from build123d import *

# Parameters (mm, degrees)
SKETCH1_R           = 42.672
SKETCH1_R_2         = 38.862
BOSS_EXTRUDE1_DEPTH = 29.21
SKETCH2_R           = 42.672
SKETCH2_R_2         = 14.478
BOSS_EXTRUDE2_DEPTH = 7.62
SKETCH3_R           = 2.159
CUT_EXTRUDE1_DEPTH  = 43.672
CIRPATTERN1_COUNT   = 4


with BuildPart() as part:
    # Sketch1 → Boss-Extrude1 (new body)
    with BuildSketch(Plane(origin=(0, 0, 0), x_dir=(1, 0, 0), z_dir=(0, 1, 0))):
        Circle(SKETCH1_R)
        Circle(SKETCH1_R_2, mode=Mode.SUBTRACT)
    extrude(amount=BOSS_EXTRUDE1_DEPTH)

    # Sketch2 → Boss-Extrude2 (add)
    with BuildSketch(Plane(origin=(0, 29.21, 0), x_dir=(1, 0, 0), z_dir=(0, 1, 0))):
        Circle(SKETCH2_R)
        Circle(SKETCH2_R_2, mode=Mode.SUBTRACT)
    extrude(amount=BOSS_EXTRUDE2_DEPTH)

    # Sketch3 → Cut-Extrude1 (cut, symmetric)
    with BuildSketch(Plane.XY):
        with Locations((0, 3.937)):
            Circle(SKETCH3_R)
    cut_extrude1 = extrude(amount=CUT_EXTRUDE1_DEPTH, both=True, mode=Mode.SUBTRACT)

    # CirPattern1: Cut-Extrude1 ×4 about axis
    cirpattern1_axis = Axis((0, 29.21, 0), (0, -1, 0))
    for i in range(1, CIRPATTERN1_COUNT):
        add(cut_extrude1.rotate(cirpattern1_axis, i * 360 / CIRPATTERN1_COUNT), mode=Mode.SUBTRACT)


solid = part.part
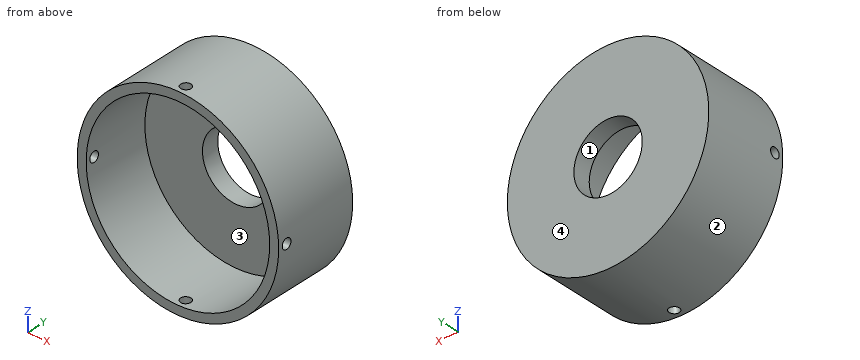
Model file for the job. Use its own axes, mm. Face numbers are marked on the shaded views. Give positions to 0.01 mm unless a question says otherwise; leave off trailing zeros. Loops run counter-clockwise (first coordinate to the right, second up) from the corner with the lowest first, then second, coordinate; pieces in that order, holes last.
1) Saw through at C-C (z = 12). Write the cut outline in (x, y), plus the area to 3 significant figures.
2) Wall check: line 1 (Y direction, x = 0, z = -39.75); line 2 (Z direction, x = 0, y = 34.5); line 3 (Z direction, x = 0, y = 22). Give the ranges that are in metal, low to high.
3) Saw through at A-A (z = 0). Write the cut outline in (x, y).
4) Flat gauge pins, fed straight in: pin 1 Ø5.5 at (x, y) = (0, 3.937) entering from -Z; pin 2 Ø10 at (x, y) = (-22, 8) entering from +Z; pin 3 Ø6 at (x, z) = (-32, -10.5) entering from -Y; pin 4 Ø8 at (x, y) = (28.5, 11) entering from +Z. Where does each tip first touch, or does it go through?
5) Pull direction X, two halves, no side cores. Call the marked faces 1, 2, 3 and 4: +X half, -X half, draft (parallel to the pull), parting line (faces both ways), or undercut.
6) Saw through at B-B (x = 0). Write the cut outline in (y, z), plus the area to 3 significant figures.
7) Saw through at D-D (y = 27.5). Write the cut outline in (x, z), plus the area to 3 significant figures.
Answer block:
1. outline: (-40.95, 0) - (-36.96, 0) - (-36.96, 29.21) - (-8.1, 29.21) - (-8.1, 36.83) - (-40.95, 36.83) - close; (8.1, 29.21) - (36.96, 29.21) - (36.96, 0) - (40.95, 0) - (40.95, 36.83) - (8.1, 36.83) - close
1. area: 734 mm2
2. line 1: y = 0 to 1.78, 6.1 to 36.83
2. line 2: z = -42.67 to -14.48, 14.48 to 42.67
2. line 3: z = -42.67 to -38.86, 38.86 to 42.67
3. outline: (-42.67, 0) - (-38.86, 0) - (-38.86, 1.78) - (-42.67, 1.78) - close; (-42.67, 6.1) - (-38.86, 6.1) - (-38.86, 29.21) - (-14.48, 29.21) - (-14.48, 36.83) - (-42.67, 36.83) - close; (14.48, 29.21) - (38.86, 29.21) - (38.86, 6.1) - (42.67, 6.1) - (42.67, 36.83) - (14.48, 36.83) - close; (38.86, 0) - (42.67, 0) - (42.67, 1.78) - (38.86, 1.78) - close
4. pin 1: stops at z = -42.67
4. pin 2: stops at z = 39.14
4. pin 3: stops at y = 29.21
4. pin 4: stops at z = 34.94
5. face 1: undercut
5. face 2: parting line
5. face 3: undercut
5. face 4: draft
6. outline: (0, -42.67) - (1.78, -42.67) - (1.78, -38.86) - (0, -38.86) - close; (0, 38.86) - (1.78, 38.86) - (1.78, 42.67) - (0, 42.67) - close; (6.1, -42.67) - (36.83, -42.67) - (36.83, -14.48) - (29.21, -14.48) - (29.21, -38.86) - (6.1, -38.86) - close; (6.1, 38.86) - (29.21, 38.86) - (29.21, 14.48) - (36.83, 14.48) - (36.83, 42.67) - (6.1, 42.67) - close
6. area: 619 mm2
7. outline: circle Ø85.34 at (0, 0); hole circle Ø77.72 at (0, 0)
7. area: 976 mm2
